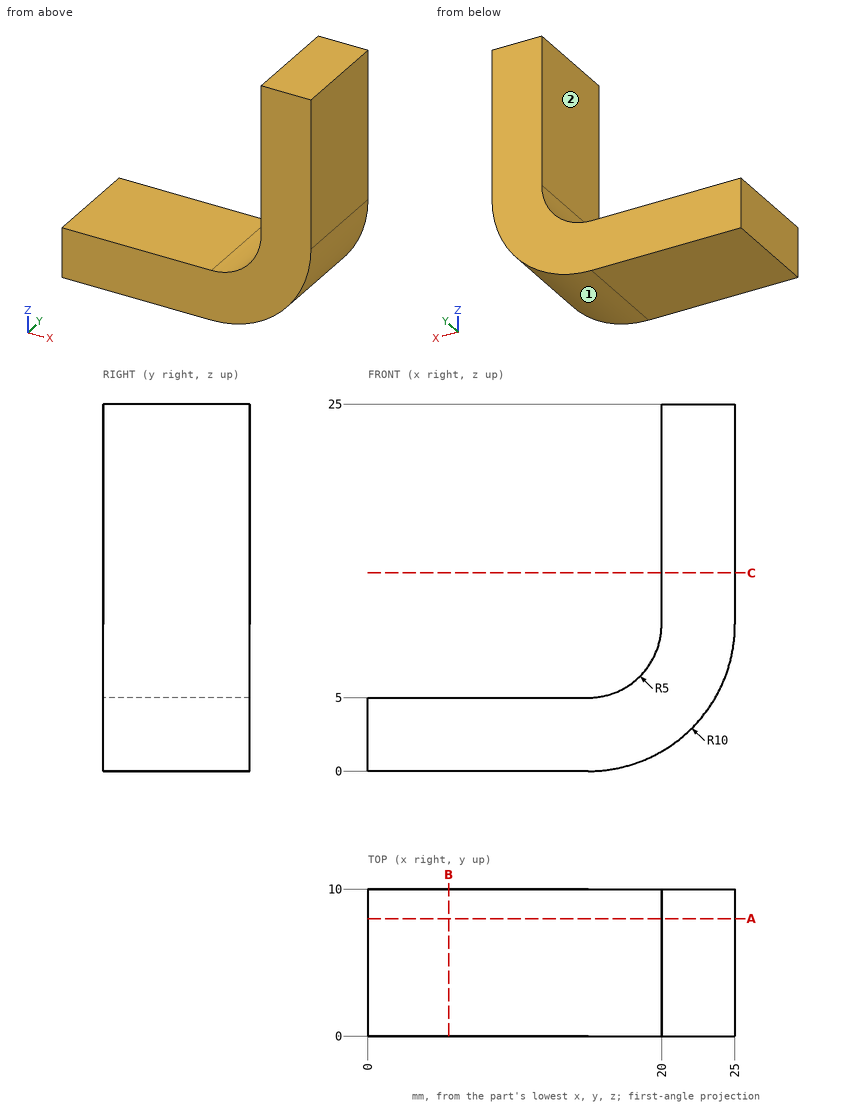
The drawing under review shows one solid part. Ordinate dimensions are in mm from its lowest x, y, z. A direction names the side the tool comes from. Coordinates: 2 decimals unless noted, no trailing zeros. Write each loop counter-clockwise with the first axis right and the second up, starting at its lowest first coordinate (ties: lowest second). Pieces come first, ordered by that corner, then holes. Notation, with made-up numbers: (-24.5, 19) - (-13.5, 19) arc R15 ccw to (-13.5, 32) - close; hole circle Ø5 at (43, -37.75). An arc over 180 degrees is marked (long way). Answer as CSV lines item,"result".
(1) For line 1 along X through (y, z) = (5.5, 18); line 2 along Z through (x, y) = (3.5, 9.25); line 3 along X through (y, z) = (2.5, 8.25), list the stretches that pass through material, from the lowest coordinate up. Write a range as [from, to].
Data:
line 1,"x = [20, 25]"
line 2,"z = [0, 5]"
line 3,"x = [19.68, 24.85]"
(2) We need section B-B (x = 5.5). Give the boundary of the cut face in (y, z), plus the area to 3 significant figures.
Data:
outline,"(0, 0) - (10, 0) - (10, 5) - (0, 5) - close"
area,"50.0 mm2"
(3) Clearance check with flat-ended pins moving along their axes: pin 1 Ø5 at (x, y) = (14.5, 9) entering from +Z; pin 2 Ø2 at (x, y) = (12.5, 1.5) entering from +Z; pin 3 Ø1 at (y, z) = (8.5, 19.5) entering from -X. State where each tip first meets the part, or that it passes through.
Data:
pin 1,"stops at z = 5.42"
pin 2,"stops at z = 5"
pin 3,"stops at x = 20"
(4) We need section C-C (z = 13.5). Give the boundary of the cut face in (x, y), plus the area to 3 significant figures.
Data:
outline,"(20, 0) - (25, 0) - (25, 10) - (20, 10) - close"
area,"50.0 mm2"
(5) We need section A-A (y = 8). Give the boundary of the cut face in (x, z).
Data:
outline,"(0, 0) - (15, 0) arc R10 ccw to (25, 10) - (25, 25) - (20, 25) - (20, 10) arc R5 cw to (15, 5) - (0, 5) - close"
(6) Tool access review of the marked faces 1 and 2: name each direction out of +Z, -Z, +X, -X, +Y, -Y from which nothing blocks a thin tool from reaching the whole face with its end or side.
Data:
face 1,"-Z, +X, +Y, -Y"
face 2,"+Z, -X, +Y, -Y"
